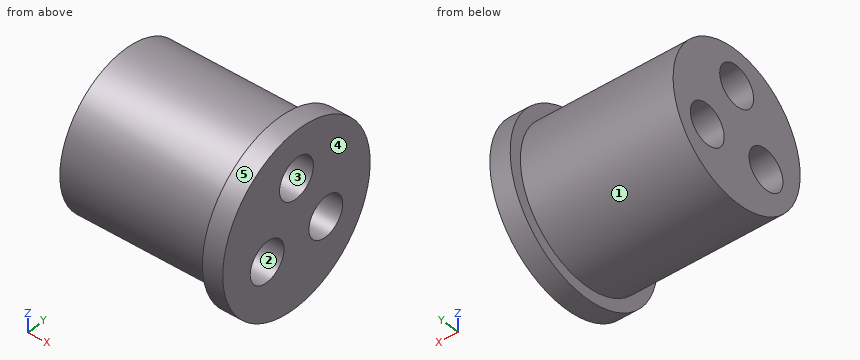
from build123d import *

# Parameters (mm, degrees)
BOSS_EXTRUDE1_OUTLINE_R   = 37.5
BOSS_EXTRUDE1_OUTLINE_R_2 = 10
BOSS_EXTRUDE1_DEPTH       = 75
SKETCH3_R                 = 43.5
SKETCH3_R_2               = 10
BOSS_EXTRUDE2_DEPTH       = 10


# Read off the part's stored shape, not the designer's step: Boss-Extrude1
with BuildPart() as part:
    # Boss-Extrude1 outline → Boss-Extrude1 (new body)
    with BuildSketch(Plane(origin=(0, 0, 0), x_dir=(0, 0, -1), z_dir=(1, 0, 0))):
        Circle(BOSS_EXTRUDE1_OUTLINE_R)
        with Locations((10, -17.320508076)):
            Circle(BOSS_EXTRUDE1_OUTLINE_R_2, mode=Mode.SUBTRACT)
        with Locations((-20, 0)):
            Circle(BOSS_EXTRUDE1_OUTLINE_R_2, mode=Mode.SUBTRACT)
        with Locations((10, 17.320508076)):
            Circle(BOSS_EXTRUDE1_OUTLINE_R_2, mode=Mode.SUBTRACT)
    extrude(amount=BOSS_EXTRUDE1_DEPTH)

    # Sketch3 → Boss-Extrude2 (add)
    with BuildSketch(Plane(origin=(75, 0, 0), x_dir=(0, 0, -1), z_dir=(1, 0, 0))):
        Circle(SKETCH3_R)
        with Locations((-20, 0)):
            Circle(SKETCH3_R_2, mode=Mode.SUBTRACT)
        with Locations((10, 17.320508076)):
            Circle(SKETCH3_R_2, mode=Mode.SUBTRACT)
        with Locations((10, -17.320508076)):
            Circle(SKETCH3_R_2, mode=Mode.SUBTRACT)
    extrude(amount=BOSS_EXTRUDE2_DEPTH)


solid = part.part
Build history of the part. All positions in model axes, mm. Face numbers are marked on the shaded views. A direction names the side the tool comes from. Coordinates: 2 decimals unless noted, no trailing zeros. Order: outer loops, then holes, each group sorted by start corner. A loop starts at its lowest first (then second) coordinate and runs counter-clockwise, first axis right, second up. Notation, with made-up numbers: (0.25, 79.25) - (24.25, 79.25) arc R14 ccw to (24.25, 93.25) - close; hole circle Ø9 at (84, -26). An arc over 180 degrees is marked (long way). Write item = value, one per line. Start each with the question number.
1) Flat gauge pins, fed straight in: pin 1 Ø12 at (y, z) = (18, -27.5) entering from -X; pin 2 Ø1 at (x, z) = (61.5, 12) entering from +Y; pin 3 Ø3 at (x, z) = (66.5, 15) entering from +Y; pin 4 Ø12 at (x, y) = (52.5, -21.5) entering from +Z. Where does each tip first touch, or does it go through?
2) 3-axis set-ups, long thin cutter, end or side, ignore diameter. For the marked faces 1 and 2: which of +Z, -Z, +X, -X, +Y, -Y reach the whole face in a straight line?
3) Two-plate mould, pull along Z, no slides. Class the marked faces 3, 4 and 5: pulls with the +Z half, pulls with the -Z half, needs draft (parallel to the pull), parting line crosses it, or undercut.
4) Saw through at C-C on z = -10. Write the cut outline in (x, y), then the cut area to 3 significant figures.
5) Wall check: line 1 along Z through (x, y) = (79, 0.5); line 2 along Y through (x, z) = (53.5, -10); line 3 along X through (y, z) = (36, -16). Give the ranges that are in metal, low to high. Write a range as from..to.
6) Saw through at B-B on z = 19.5. Write the cut outline in (x, y).
7) Saw through at D-D on x = 59. Write the cut outline in (y, z).
8) Saw through at A-A on y = 0. Write the cut outline in (x, z), then the cut area to 4 significant figures.
From the geometry:
q1.pin_1 = 0
q1.pin_2 = 35.69
q1.pin_3 = 34.99
q1.pin_4 = 34.15
q2.face_1 = -X
q2.face_2 = +X, -X
q3.face_3 = undercut
q3.face_4 = needs draft
q3.face_5 = parting line crosses it
q4.outline = (0, -36.14) - (75, -36.14) - (75, -42.33) - (85, -42.33) - (85, -27.32) - (0, -27.32) - close; (0, -7.32) - (85, -7.32) - (85, 7.32) - (0, 7.32) - close; (0, 27.32) - (85, 27.32) - (85, 42.33) - (75, 42.33) - (75, 36.14) - (0, 36.14) - close
q4.area = 2,870 mm^2
q5.line_1 = -43.5..10.01, 29.99..43.5
q5.line_2 = -36.14..-27.32, -7.32..7.32, 27.32..36.14
q5.line_3 = 75..85
q6.outline = (0, -32.03) - (75, -32.03) - (75, -38.88) - (85, -38.88) - (85, -9.99) - (0, -9.99) - close; (0, 9.99) - (85, 9.99) - (85, 38.88) - (75, 38.88) - (75, 32.03) - (0, 32.03) - close
q7.outline = circle Ø75 at (0, 0); hole circle Ø20 at (-17.32, -10); hole circle Ø20 at (0, 20); hole circle Ø20 at (17.32, -10)
q8.outline = (0, -37.5) - (75, -37.5) - (75, -43.5) - (85, -43.5) - (85, 10) - (0, 10) - close; (0, 30) - (85, 30) - (85, 43.5) - (75, 43.5) - (75, 37.5) - (0, 37.5) - close
q8.area = 4,795 mm^2
